The model under review builds one solid part; all positions refer to its coordinate system, in mm. A direction names the side the tool comes from. Coordinates: 2 decimals unless noted, no trailing zeros. Order: outer loops, then holes, each group sorted by start corner. A loop starts at its lowest first (then second) coordinate and runs counter-clockwise, first axis right, second up. Notation, with made-up numbers: (75, 5.25) -> (114, 5.25) arc R24 cw to (114, 39.25) -> close; hole circle Ø3 at (53, 78). An arc over 180 degrees is marked (long way). Use one line per item in the form item = value.
from build123d import *

# Parameters (mm, degrees)
REVOLVE1_ANGLE                  = 180
BOSS_EXTRUDE2_DEPTH             = 4
BOSS_EXTRUDE4_DEPTH             = 3
SKETCH12_R                      = 4
BOSS_EXTRUDE5_DEPTH             = 2
CUT_EXTRUDE2_REACH              = 100.408
SKETCH13_R                      = 1.25
SKETCH14_R                      = 3.5
SKETCH14_R_2                    = 2.05
CUT_EXTRUDE3_DEPTH              = 0.75
F_1_4_0_25_DIAMETER_HOLE1_D     = 6.35
F_1_4_0_25_DIAMETER_HOLE1_DEPTH = 4
F_1_4_0_25_DIAMETER_HOLE1_TIP   = 1.907732465


with BuildPart() as part:
    # Sketch2 → Revolve1 (revolve)
    with BuildSketch(Plane(origin=(0, 0, 0), x_dir=(1, 0, 0), z_dir=(0, 1, 0))):
        with BuildLine():
            Line((79.585159762, 39.800683112), (74.585159762, 39.800683112))
            ThreePointArc((74.585159762, 39.800683112), (71.049625856, 38.336217018), (69.585159762, 34.800683112))
            Line((69.585159762, 34.800683112), (71.085159762, 34.800683112))
            ThreePointArc((71.085159762, 34.800683112), (72.110286027, 37.275556846), (74.585159762, 38.300683112))
            Line((74.585159762, 38.300683112), (79.585159762, 38.300683112))
            ThreePointArc((79.585159762, 38.300683112), (82.060033496, 37.275556846), (83.085159762, 34.800683112))
            Line((83.085159762, 34.800683112), (84.585159762, 34.800683112))
            ThreePointArc((84.585159762, 34.800683112), (83.120693668, 38.336217018), (79.585159762, 39.800683112))
        make_face()
    revolve(axis=Axis((74.585159762, 0, -34.800683112), (-1, 0, 0)), revolution_arc=REVOLVE1_ANGLE)

    # Sketch7 → Boss-Extrude2 (add)
    with BuildSketch(Plane(origin=(0, 0, 0), x_dir=(1, 0, 0), z_dir=(0, 1, 0))):
        with BuildLine():
            Line((74.585159762, 39.800683112), (79.585159762, 39.800683112))
            ThreePointArc((79.585159762, 39.800683112), (83.120693668, 38.336217018), (84.585159762, 34.800683112))
            ThreePointArc((84.585159762, 34.800683112), (83.120693668, 31.265149206), (79.585159762, 29.800683112))
            Line((79.585159762, 29.800683112), (74.585159762, 29.800683112))
            ThreePointArc((74.585159762, 29.800683112), (71.049625856, 31.265149206), (69.585159762, 34.800683112))
            ThreePointArc((69.585159762, 34.800683112), (71.049625856, 38.336217018), (74.585159762, 39.800683112))
        make_face()
        with BuildLine():
            Line((74.585159762, 38.300683112), (79.585159762, 38.300683112))
            ThreePointArc((79.585159762, 38.300683112), (82.060033496, 37.275556846), (83.085159762, 34.800683112))
            ThreePointArc((83.085159762, 34.800683112), (82.060033496, 32.325809378), (79.585159762, 31.300683112))
            Line((79.585159762, 31.300683112), (74.585159762, 31.300683112))
            ThreePointArc((74.585159762, 31.300683112), (72.110286027, 32.325809378), (71.085159762, 34.800683112))
            ThreePointArc((71.085159762, 34.800683112), (72.110286027, 37.275556846), (74.585159762, 38.300683112))
        make_face(mode=Mode.SUBTRACT)
    extrude(amount=BOSS_EXTRUDE2_DEPTH)

    # Sketch8 → Boss-Extrude4 (add)
    with BuildSketch(Plane(origin=(0, 4, 0), x_dir=(1, 0, 0), z_dir=(0, 1, 0))):
        with BuildLine():
            Line((86.285159762, 45.200683112), (67.885159762, 45.200683112))
            Line((67.885159762, 45.200683112), (67.885159762, 42.180683112))
            Line((67.885159762, 42.180683112), (81.625159762, 42.180683112))
            ThreePointArc((81.625159762, 42.180683112), (83.125159762, 43.680683112), (84.625159762, 42.180683112))
            ThreePointArc((84.625159762, 42.180683112), (84.185819933, 41.12002294), (83.125159762, 40.680683112))
            Line((83.125159762, 40.680683112), (83.125159762, 38.331745275))
            ThreePointArc((83.125159762, 38.331745275), (84.585159762, 34.800683112), (83.125159762, 31.269620949))
            Line((83.125159762, 31.269620949), (83.125159762, 24.400683112))
            Line((83.125159762, 24.400683112), (86.285159762, 24.400683112))
            Line((86.285159762, 24.400683112), (86.285159762, 45.200683112))
        make_face()
        with BuildLine():
            Line((81.625159762, 42.180683112), (67.885159762, 42.180683112))
            Line((67.885159762, 42.180683112), (67.885159762, 34.560683112))
            Line((67.885159762, 34.560683112), (69.590923083, 34.560683112))
            ThreePointArc((69.590923083, 34.560683112), (70.965767547, 38.250320774), (74.585159762, 39.800683112))
            Line((74.585159762, 39.800683112), (79.585159762, 39.800683112))
            ThreePointArc((79.585159762, 39.800683112), (81.501496004, 39.418870571), (83.125159762, 38.331745275))
            Line((83.125159762, 38.331745275), (83.125159762, 40.680683112))
            ThreePointArc((83.125159762, 40.680683112), (82.06449959, 41.12002294), (81.625159762, 42.180683112))
        make_face()
        with BuildLine():
            ThreePointArc((74.585159762, 39.800683112), (70.965767547, 38.250320774), (69.590923083, 34.560683112))
            Line((69.590923083, 34.560683112), (71.093398029, 34.560683112))
            ThreePointArc((71.093398029, 34.560683112), (72.02684, 37.189197295), (74.585159762, 38.300683112))
            Line((74.585159762, 38.300683112), (79.585159762, 38.300683112))
            ThreePointArc((79.585159762, 38.300683112), (83.085159762, 34.800683112), (79.585159762, 31.300683112))
            Line((79.585159762, 31.300683112), (79.315159762, 31.300683112))
            Line((79.315159762, 31.300683112), (79.315159762, 29.800683112))
            Line((79.315159762, 29.800683112), (79.585159762, 29.800683112))
            ThreePointArc((79.585159762, 29.800683112), (81.501496004, 30.182495653), (83.125159762, 31.269620949))
            Line((83.125159762, 31.269620949), (83.125159762, 38.331745275))
            ThreePointArc((83.125159762, 38.331745275), (81.501496004, 39.418870571), (79.585159762, 39.800683112))
            Line((79.585159762, 39.800683112), (74.585159762, 39.800683112))
        make_face()
        with BuildLine():
            Line((83.125159762, 38.331745275), (83.125159762, 31.269620949))
            ThreePointArc((83.125159762, 31.269620949), (84.585159762, 34.800683112), (83.125159762, 38.331745275))
        make_face()
        with BuildLine():
            ThreePointArc((74.585159762, 38.300683112), (72.02684, 37.189197295), (71.093398029, 34.560683112))
            Line((71.093398029, 34.560683112), (79.315159762, 34.560683112))
            Line((79.315159762, 34.560683112), (79.315159762, 31.300683112))
            Line((79.315159762, 31.300683112), (79.585159762, 31.300683112))
            ThreePointArc((79.585159762, 31.300683112), (83.085159762, 34.800683112), (79.585159762, 38.300683112))
            Line((79.585159762, 38.300683112), (74.585159762, 38.300683112))
        make_face()
        with BuildLine():
            Line((71.093398029, 34.560683112), (69.590923083, 34.560683112))
            ThreePointArc((69.590923083, 34.560683112), (71.135522099, 31.181290898), (74.585159762, 29.800683112))
            Line((74.585159762, 29.800683112), (79.315159762, 29.800683112))
            Line((79.315159762, 29.800683112), (79.315159762, 31.300683112))
            Line((79.315159762, 31.300683112), (74.585159762, 31.300683112))
            ThreePointArc((74.585159762, 31.300683112), (72.196645579, 32.242363351), (71.093398029, 34.560683112))
        make_face()
        with BuildLine():
            Line((79.315159762, 34.560683112), (71.093398029, 34.560683112))
            ThreePointArc((71.093398029, 34.560683112), (72.196645579, 32.242363351), (74.585159762, 31.300683112))
            Line((74.585159762, 31.300683112), (79.315159762, 31.300683112))
            Line((79.315159762, 31.300683112), (79.315159762, 34.560683112))
        make_face()
        with BuildLine():
            Line((74.005159762, 26.940683112), (67.885159762, 26.940683112))
            Line((67.885159762, 26.940683112), (67.885159762, 24.400683112))
            Line((67.885159762, 24.400683112), (75.505159762, 24.400683112))
            Line((75.505159762, 24.400683112), (75.505159762, 25.440683112))
            ThreePointArc((75.505159762, 25.440683112), (74.44449959, 25.88002294), (74.005159762, 26.940683112))
        make_face()
        with BuildLine():
            Line((79.315159762, 24.400683112), (83.125159762, 24.400683112))
            Line((83.125159762, 24.400683112), (83.125159762, 31.269620949))
            ThreePointArc((83.125159762, 31.269620949), (81.501496004, 30.182495653), (79.585159762, 29.800683112))
            Line((79.585159762, 29.800683112), (79.315159762, 29.800683112))
            Line((79.315159762, 29.800683112), (79.315159762, 24.400683112))
        make_face()
        with BuildLine():
            Line((69.590923083, 34.560683112), (67.885159762, 34.560683112))
            Line((67.885159762, 34.560683112), (67.885159762, 26.940683112))
            Line((67.885159762, 26.940683112), (74.005159762, 26.940683112))
            ThreePointArc((74.005159762, 26.940683112), (75.505159762, 28.440683112), (77.005159762, 26.940683112))
            ThreePointArc((77.005159762, 26.940683112), (76.565819933, 25.88002294), (75.505159762, 25.440683112))
            Line((75.505159762, 25.440683112), (75.505159762, 24.400683112))
            Line((75.505159762, 24.400683112), (79.315159762, 24.400683112))
            Line((79.315159762, 24.400683112), (79.315159762, 29.800683112))
            Line((79.315159762, 29.800683112), (74.585159762, 29.800683112))
            ThreePointArc((74.585159762, 29.800683112), (71.135522099, 31.181290898), (69.590923083, 34.560683112))
        make_face()
    extrude(amount=BOSS_EXTRUDE4_DEPTH)

    # Sketch12 → Boss-Extrude5 (add)
    with BuildSketch(Plane(origin=(0, 7, 0), x_dir=(1, 0, 0), z_dir=(0, 1, 0))):
        with Locations(Location((79.315159762, 34.560683112, 0), (0, 0, 270))):
            Circle(SKETCH12_R)
    extrude(amount=BOSS_EXTRUDE5_DEPTH)

    # Sketch13 → Cut-Extrude2 (cut, up to next)
    with BuildSketch(Plane(origin=(0, 9, 0), x_dir=(1, 0, 0), z_dir=(0, 1, 0)), mode=Mode.PRIVATE) as cut_extrude2_sk1:
        with Locations(Location((79.315159762, 34.560683112, 0), (0, 0, 270))):
            Circle(SKETCH13_R)
    cut_extrude2_tool1 = extrude(cut_extrude2_sk1.sketch, amount=-CUT_EXTRUDE2_REACH, mode=Mode.PRIVATE) & part.part
    add(cut_extrude2_tool1.solids().sort_by_distance((79.31516, 9, -34.560683))[0], mode=Mode.SUBTRACT)

    # Sketch14 → Cut-Extrude3 (cut)
    with BuildSketch(Plane(origin=(0, 9, 0), x_dir=(1, 0, 0), z_dir=(0, 1, 0))):
        with Locations(Location((79.315159762, 34.560683112, 0), (0, 0, 270))):
            Circle(SKETCH14_R)
        with Locations(Location((79.315159762, 34.560683112, 0), (0, 0, 270))):
            Circle(SKETCH14_R_2, mode=Mode.SUBTRACT)
    extrude(amount=-CUT_EXTRUDE3_DEPTH, mode=Mode.SUBTRACT)

    # 1/4 (0.25) Diameter Hole1
    with Locations(Plane(origin=(77.057625156, -5, -34.800683112), x_dir=(0, 0, -1), z_dir=(0, -1, 0))):
        with Locations((0, 0)):
            Hole(F_1_4_0_25_DIAMETER_HOLE1_D / 2, depth=F_1_4_0_25_DIAMETER_HOLE1_DEPTH)
            with Locations((0, 0, -(F_1_4_0_25_DIAMETER_HOLE1_DEPTH + F_1_4_0_25_DIAMETER_HOLE1_TIP / 2))):  # 118° drill point
                Cone(0, F_1_4_0_25_DIAMETER_HOLE1_D / 2, F_1_4_0_25_DIAMETER_HOLE1_TIP, mode=Mode.SUBTRACT)


solid = part.part
Item 1: To check wall thickness, follow L1, parallel to X at y = 2.75, z = -35; L2, parallel to Z at x = 78.25, y = 2; L3, parallel to Y at x = 70.5, z = -27.5. State the ranges of each line that lie inside material, in increasing order. Write a range as from..to.
Results found:
L1 = 69.59..71.09, 83.08..84.58
L2 = -39.8..-38.3, -31.3..-29.8
L3 = 4..7
Item 2: We need section C-C (z = -42.5). Write out the cut boundary in (x, y).
Results found:
outline = (67.89, 4) -> (81.66, 4) -> (81.66, 7) -> (67.89, 7) -> close; (84.59, 4) -> (86.29, 4) -> (86.29, 7) -> (84.59, 7) -> close
Item 3: Tool access review of faces 5 (the face through (77, 8.25, -35)), 6 (the face through (77, 2, -39.801)), 7 (the face through (77.12, -0.973, -31.439)): name each direction out of +Z, -Z, +X, -X, +Y, -Y from which nothing blocks a thin tool from reaching the whole face with its end or side.
Results found:
face_5 = +Y
face_6 = -Z, +X, -X, -Y
face_7 = none
Item 4: We need section D-D (x = 72). Write out the cut boundary in (y, z), plus the area to 3 significant figures.
Results found:
outline = (0, -39.08) -> (4, -39.08) -> (4, -45.2) -> (7, -45.2) -> (7, -24.4) -> (4, -24.4) -> (4, -30.52) -> (0, -30.52) arc R4.28 ccw to start; hole (0, -37.16) -> (4, -37.16) -> (4, -32.44) -> (0, -32.44) arc R2.36 ccw to start
area = 97.8 mm²
Item 5: Draft analysis for pull direction Y (two halves, no side actions). For faces 1 (the face through (77.12, -0.927, -38.176)), 2 (the face through (77, 2, -38.301)), 3 (the face through (79, 9, -33)), 4 (the face through (77, 2, -29.801)), state which applies: released by +Y, released by -Y, zero draft, split by the parting line, or undercut.
Results found:
face_1 = undercut
face_2 = undercut
face_3 = released by +Y
face_4 = zero draft
Item 6: We need section A-A (y = 1.5). Write out the cut boundary in (x, z), plus the area to 3 significant figures.
Results found:
outline = (74.59, -39.8) -> (79.59, -39.8) arc R5 ccw to (79.59, -29.8) -> (74.59, -29.8) arc R5 ccw to start; hole (74.59, -38.3) -> (79.59, -38.3) arc R3.5 ccw to (79.59, -31.3) -> (74.59, -31.3) arc R3.5 ccw to start
area = 55.1 mm²
Item 7: Clearance check with flat-ended pins moving along their axes: pin 1 (1 mm diameter, centred on y = -1.5, z = -34.5, fed in from -X); pin 2 (1.2 mm diameter, centred on x = 77.5, y = 2, fed in from +Z); pin 3 (2 mm diameter, centred on x = 75, z = -35, fed in from -Y); pin 4 (11 mm diameter, centred on x = 79.32, z = -34.56, fed in from -Y). State where each tip first meets the part, or that it passes through.
Results found:
pin_1 = 69.69
pin_2 = -29.8
pin_3 = 4
pin_4 = -4.96
